Part model, mm, in its own coordinate system. Round coordinates to 2 decimals unless told otherwise and drop trailing zeros. Order: outer loops, then holes, each group sorted by start corner. A loop starts at its lowest first (then second) coordinate and runs counter-clockwise, first axis right, second up. Notation, with made-up numbers: (70.5, 79) - (123.5, 79) arc R32 ccw to (123.5, 118) - close; hole circle Ø7 at (62, -36). An arc over 180 degrees is marked (long way). Answer as a JSON object with one key per item and string values.
Solid Edge part; units mm, degrees
sketch "Sketch1" plane through (0, 0, 0) normal (0, -1, 0) x (1, 0, 0)
  line L0 (0, 0) -> (0, 1240)
  line L1 (0, 1240) -> (-600, 1240)
  line L2 (-600, 1240) -> (-1900, 920)
  line L3 (-1900, 0) -> (-1900, 920)
sketch "Sketch2" plane through (0, 0, 0) normal (0, 0, 1) x (1, 0, 0)
  circle A0 centre (0, 0) radius 16.85
sweep "SweptProtrusion_1" add profiles "Sketch2" path "Sketch1"
sketch "Sketch3" plane through (0, 0, 0) normal (0, 0, 1) x (1, 0, 0)
  line L0 (-1916.85, 16.7) -> (-1846.85, 16.7)
  line L1 (-1846.85, 16.7) -> (-1846.85, -23.3)
  line L2 (-1846.85, -23.3) -> (-1916.85, -23.3)
  line L3 (-1916.85, -23.3) -> (-1916.85, 16.7)
  line L4 (-655, 16.7) -> (-545, 16.7)
  line L5 (-545, 16.7) -> (-545, -23.3)
  line L6 (-545, -23.3) -> (-655, -23.3)
  line L7 (-655, -23.3) -> (-655, 16.7)
  line L8 (-53.15, -23.15) -> (16.85, -23.15)
  line L9 (16.85, 16.85) -> (16.85, -23.15)
  line L10 (16.85, 16.85) -> (-53.15, 16.85)
  line L11 (-53.15, 16.85) -> (-53.15, -23.15)
  dimension "D1" = 16.85
  dimension "D2" = 1846.85
  dimension "D3" = 545
  dimension "D4" = 655
  dimension "D5" = 16.85
  dimension "D6" = 1846.85
extrude "ExtrudedProtrusion_1" add sketch "Sketch3" along normal blind 3.18
sketch "Sketch4" plane through (0, 0, 0) normal (0, 0, 1) x (1, 0, 0)
  circle A0 centre (-600, 0) radius 16.7
extrude "Protrusion1" add sketch "Sketch4" along normal up to vertex (1240 mm away)
sketch "Sketch5" plane through (0, 0, 0) normal (0, -1, 0) x (1, 0, 0)
  line L0 (0, 780) -> (-600, 780)
  line L1 (-600, 780) -> (-1900, 460)
sketch "Sketch6" plane through (0, 0, 780) normal (1, 0, 0) x (0, 1, 0)
  circle A0 centre (0, 0) radius 10.65
sweep "SweptProtrusion_2" add profiles "Sketch6" path "Sketch5"
sketch "Sketch7" plane through (-600, -3.3, 0) normal (0, 0, -1) x (1, 0, 0)
  circle A0 centre (-40, 0) radius 5
  circle A1 centre (40, 0) radius 5
  circle A2 centre (-1261.85, 0) radius 5
  circle A3 centre (561.85, -0.15) radius 5
  dimension "D1" = 40
extrude "Cutout1" cut sketch "Sketch7" against normal up to next
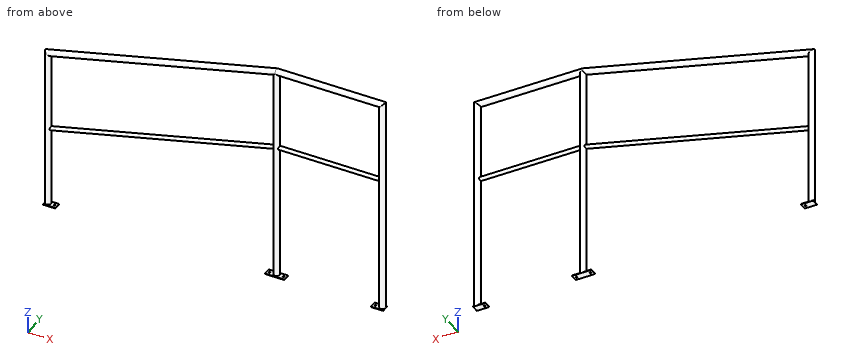
Item 1: Probe L1, parallel to X at y = 1.5, z = 190; L2, parallel to Y at x = -560, z = 2; L3, parallel to X at y = 13.5, z = 52. List the from-to ranges inside material, lowest first. Write a range as from..to.
Taken from the geometry:
{"L1": "-1916.78..-1883.22, -616.63..-583.37, -16.78..16.78", "L2": "-23.3..-8.3, 1.7..16.7", "L3": "-1910.08..-1889.92, -609.83..-590.17, -10.08..10.08"}
Item 2: Drop flat-ended pins along their axis: P1, Ø8, axis at x = -1320.5, y = 10, coming from the +Z side; P2, Ø3.5, axis at x = -29.5, z = 1.5, coming from the -Y side; P3, Ø12, axis at x = -819.5, y = -6.5, coming from the +Z side; P4, Ø16, axis at x = -560, y = -3.3, coming from the +Z side. Give the stop position or say it passes through.
Taken from the geometry:
{"P1": "z = 1079.13", "P2": "y = -23.15", "P3": "z = 1204.24", "P4": "z = 1256.85"}
Item 3: Cut at B-B (x = -116). Write the cut outline in (y, z), plus the area to 3 significant figures.
Taken from the geometry:
{"outline": "circle Ø33.7 at (0, 1240); circle Ø21.3 at (0, 780)", "area": "1,250 mm2"}
